Job drawing, mm, ordinate dimensions from the low corner. One solid piece. A direction names the side the tool comes from. Round coordinates to 2 decimals unless told otherwise and drop trailing zeros. Loops run counter-clockwise (first coordinate to the right, second up) from the corner with the lowest first, then second, coordinate; pieces in that order, holes last.
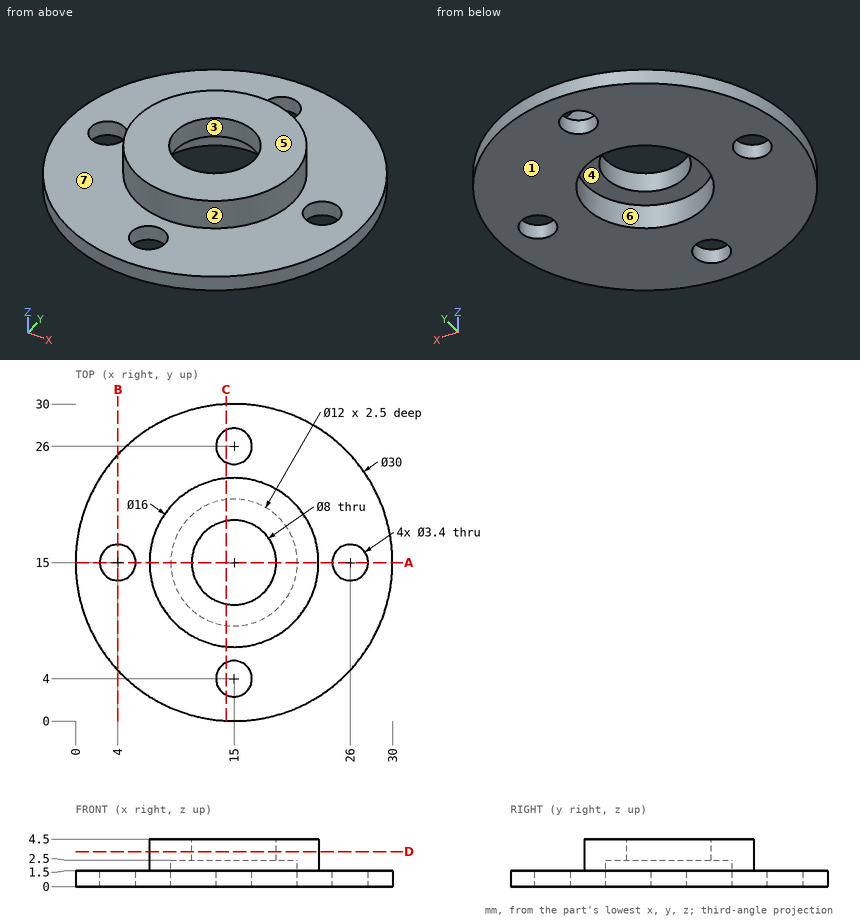
(1) Slice it at C-C on x = 14.25. List the corners of the cut face in (y, z).
Responses:
outline: (0.02, 0) - (2.47, 0) - (2.47, 1.5) - (0.02, 1.5) - close; (5.53, 0) - (9.05, 0) - (9.05, 2.5) - (11.07, 2.5) - (11.07, 4.5) - (7.04, 4.5) - (7.04, 1.5) - (5.53, 1.5) - close; (18.93, 2.5) - (20.95, 2.5) - (20.95, 0) - (24.47, 0) - (24.47, 1.5) - (22.96, 1.5) - (22.96, 4.5) - (18.93, 4.5) - close; (27.53, 0) - (29.98, 0) - (29.98, 1.5) - (27.53, 1.5) - close
(2) Which spindle directions (+Z, -Z, +X, -X, +Y, -Y) get a long thin tool onto all of the face, cutting with end or side? Do the marked faces 5, 6 and 7. Say none if no direction does.
Responses:
face 5: +Z, +X, -X, +Y, -Y
face 6: -Z
face 7: +Z
(3) Slice it at A-A on y = 15. List the corners of the cut face in (x, z), plus the area to 3 significant figures.
Responses:
outline: (0, 0) - (2.3, 0) - (2.3, 1.5) - (0, 1.5) - close; (5.7, 0) - (9, 0) - (9, 2.5) - (11, 2.5) - (11, 4.5) - (7, 4.5) - (7, 1.5) - (5.7, 1.5) - close; (19, 2.5) - (21, 2.5) - (21, 0) - (24.3, 0) - (24.3, 1.5) - (23, 1.5) - (23, 4.5) - (19, 4.5) - close; (27.7, 0) - (30, 0) - (30, 1.5) - (27.7, 1.5) - close
area: 36.8 mm2
(4) Pull direction Y, two halves, no side cores. Call the marked faces 1, 2, 3 and 4: +Y half, -Y half, draft (parallel to the pull), parting line (faces both ways), or undercut.
Responses:
face 1: draft
face 2: parting line
face 3: undercut
face 4: undercut
(5) Slice it at D-D on z = 3.3. List the corners of the cut face in (x, y), plus the area to 3 significant figures.
Responses:
outline: circle Ø16 at (15, 15); hole circle Ø8 at (15, 15)
area: 151 mm2
(6) Pin check, flat tips, straight feed: P1, Ø3, axis at x = 4, y = 15, coming from the +Z side; P2, Ø2, axis at y = 17.5, z = 2, coming from the -X side; P3, Ø10.5, axis at x = 15, y = 15, coming from the -Z side; P4, Ø8, axis at x = 19.5, y = 27, coming from the +Z side. Stop position of each tip, or through.
Responses:
P1: passes through
P2: stops at x = 0.09
P3: stops at z = 2.5
P4: stops at z = 1.5
(7) Probe line 1 (Y direction, x = 15, z = 3.2); line 2 (Z direction, x = 14, y = 23); line 3 (Y direction, x = 17.5, z = 3.4). List the from-to ranges inside material, lowest first.
Responses:
line 1: y = 7 to 11, 19 to 23
line 2: z = 0 to 1.5
line 3: y = 7.4 to 11.88, 18.12 to 22.6
(8) Slice it at B-B on x = 4. List the corners of the cut face in (y, z), plus the area to 3 significant figures.
Responses:
outline: (4.8, 0) - (13.3, 0) - (13.3, 1.5) - (4.8, 1.5) - close; (16.7, 0) - (25.2, 0) - (25.2, 1.5) - (16.7, 1.5) - close
area: 25.5 mm2
